The model under review builds one solid part; all positions refer to its coordinate system, in mm. A direction names the side the tool comes from. Round coordinates to 2 decimals unless told otherwise and drop trailing zeros. Write each loop counter-clockwise with the first axis right and the second up, starting at its lowest first coordinate (ties: lowest second). Pieces come first, ordered by that corner, then holes. Notation, with made-up numbers: (55.5, 37) - (108.5, 37) arc R13 cw to (108.5, 44) - close; hole circle Ø5 at (9.5, 76). An arc over 180 degrees is marked (long way). Use one line per item in the form item = value.
from build123d import *

# Parameters (mm, degrees)
SKETCH1_R           = 1.5875
BOSS_EXTRUDE1_DEPTH = 60
SKETCH2_R           = 1.5875
SKETCH2_R_2         = 1.4224
CUT_EXTRUDE1_DEPTH  = 4
SKETCH7_R           = 1.5875
SKETCH7_R_2         = 1.4224
CUT_EXTRUDE2_DEPTH  = 12


with BuildPart() as part:
    # Sketch1 → Boss-Extrude1 (new body)
    with BuildSketch(Plane(origin=(0, 0, 0), x_dir=(1, 0, 0), z_dir=(0, 1, 0))):
        Circle(SKETCH1_R)
    extrude(amount=BOSS_EXTRUDE1_DEPTH)

    # Sketch2 → Cut-Extrude1 (cut)
    with BuildSketch(Plane.XZ):
        Circle(SKETCH2_R)
        Circle(SKETCH2_R_2, mode=Mode.SUBTRACT)
    extrude(amount=-CUT_EXTRUDE1_DEPTH, mode=Mode.SUBTRACT)

    # Sketch7 → Cut-Extrude2 (cut)
    with BuildSketch(Plane(origin=(0, 60, 0), x_dir=(1, 0, 0), z_dir=(0, 1, 0))):
        Circle(SKETCH7_R)
        Circle(SKETCH7_R_2, mode=Mode.SUBTRACT)
    extrude(amount=-CUT_EXTRUDE2_DEPTH, mode=Mode.SUBTRACT)


solid = part.part
(1) Add section C-C on y = 11. Write out the cut boundary in (x, z) (1 decimal), then the cut area to 3 significant figures.
Geometry results:
outline = circle Ø3.2 at (0, 0)
area = 7.92 mm2
(2) To check wall thickness, follow L1, parallel to Z at x = 0.15, y = 52; L2, parallel to X at y = 10.5, z = -0.7; L3, parallel to Y at x = -1, z = 1.1. State the ranges of each line that lie inside material, in increasing order.
Geometry results:
L1 = -1.41 to 1.41
L2 = -1.42 to 1.42
L3 = 4 to 48
(3) The part is to be moulded in two halves that separate along Y. For faces 3 (the flat face through (0, 0, 0)), 4 (the flat face through (0, 60, 0)), 5 (the cylindrical face through (-0.34, 25.69, 1.55)), say which applies: +Y half, -Y half, draft (parallel to the pull), parting line (faces both ways), or undercut.
Geometry results:
face_3 = -Y half
face_4 = +Y half
face_5 = draft
(4) Add section B-B on x = 0. Write out the cut boundary in (y, z).
Geometry results:
outline = (0, -1.42) - (4, -1.42) - (4, -1.59) - (48, -1.59) - (48, -1.42) - (60, -1.42) - (60, 1.42) - (48, 1.42) - (48, 1.59) - (4, 1.59) - (4, 1.42) - (0, 1.42) - close
(5) Add section A-A on z = 0. Write out the cut boundary in (x, y), then the cut area to 3 significant figures.
Geometry results:
outline = (-1.59, 4) - (-1.42, 4) - (-1.42, 0) - (1.42, 0) - (1.42, 4) - (1.59, 4) - (1.59, 48) - (1.42, 48) - (1.42, 60) - (-1.42, 60) - (-1.42, 48) - (-1.59, 48) - close
area = 185 mm2
(6) Machinability: for faces 1 (the cylindrical face through (-0.31, 54.08, 1.39)), 2 (the cylindrical face through (-0.31, 1.97, -1.39)), which of the approach directions +Z, -Z, +X, -X, +Y, -Y give a long, thin tool a straight path to every point of the face, cutting with its end or side? Answer none if there is none.
Geometry results:
face_1 = +Y
face_2 = -Y
(7) Insertion check: P1, Ø1, axis at x = -1, z = -1.5, coming from the -Y side; P2, Ø1, axis at x = 1, y = 46.5, coming from the -Z side. Each pin has a flat end and moves straight along its axis. Give the tip position at first contact, or say it passes through.
Geometry results:
P1 = 0
P2 = -1.51
